```python
from build123d import *

# Parameters (mm, degrees)
SKETCH1_W           = 450
SKETCH1_H           = 45
BOSS_EXTRUDE1_DEPTH = 2
SKETCH2_R           = 1.5
CUT_EXTRUDE1_DEPTH  = 227.131046077
SKETCH3_R           = 2.5
CUT_EXTRUDE2_DEPTH  = 227.131046077
SKETCH4_R           = 10
CUT_EXTRUDE3_DEPTH  = 10


with BuildPart() as part:
    # Sketch1 → Boss-Extrude1 (new body)
    with BuildSketch(Plane.XY):
        Rectangle(SKETCH1_W, SKETCH1_H)
    extrude(amount=BOSS_EXTRUDE1_DEPTH)

    # Sketch2 → Cut-Extrude1 (cut, through all)
    with BuildSketch(Plane.XY.offset(2)):
        with Locations((-50.0375, -8.55)):
            Circle(SKETCH2_R)
        with Locations((-25.0375, -8.55)):
            Circle(SKETCH2_R)
        with Locations((-11.2375, -8.55)):
            Circle(SKETCH2_R)
        with Locations((13.7625, -8.55)):
            Circle(SKETCH2_R)
        with Locations((27.5625, -8.55)):
            Circle(SKETCH2_R)
        with Locations((52.5625, -8.55)):
            Circle(SKETCH2_R)
        with Locations((-88.8375, -8.55)):
            Circle(SKETCH2_R)
        with Locations((-63.8375, -8.55)):
            Circle(SKETCH2_R)
        with BuildLine():
            Line((-31.6625, -14.4), (-45.9375, -14.4))
            ThreePointArc((-45.9375, -14.4), (-46.644606781, -14.107106781), (-46.9375, -13.4))
            Line((-46.9375, -13.4), (-46.9375, -3.7))
            ThreePointArc((-46.9375, -3.7), (-46.586028137, -2.851471863), (-45.7375, -2.5))
            Line((-45.7375, -2.5), (-31.8625, -2.5))
            ThreePointArc((-31.8625, -2.5), (-29.22852724, -3.59102724), (-28.1375, -6.225))
            Line((-28.1375, -6.225), (-28.1375, -10.875))
            ThreePointArc((-28.1375, -10.875), (-29.169948596, -13.367551404), (-31.6625, -14.4))
        make_face()
        with BuildLine():
            Line((7.1375, -14.4), (-7.1375, -14.4))
            ThreePointArc((-7.1375, -14.4), (-7.844606781, -14.107106781), (-8.1375, -13.4))
            Line((-8.1375, -13.4), (-8.1375, -3.7))
            ThreePointArc((-8.1375, -3.7), (-7.786028137, -2.851471863), (-6.9375, -2.5))
            Line((-6.9375, -2.5), (6.9375, -2.5))
            ThreePointArc((6.9375, -2.5), (9.57147276, -3.59102724), (10.6625, -6.225))
            Line((10.6625, -6.225), (10.6625, -10.875))
            ThreePointArc((10.6625, -10.875), (9.630051404, -13.367551404), (7.1375, -14.4))
        make_face()
        with BuildLine():
            Line((45.9375, -14.4), (31.6625, -14.4))
            ThreePointArc((31.6625, -14.4), (30.955393219, -14.107106781), (30.6625, -13.4))
            Line((30.6625, -13.4), (30.6625, -3.7))
            ThreePointArc((30.6625, -3.7), (31.013971863, -2.851471863), (31.8625, -2.5))
            Line((31.8625, -2.5), (45.7375, -2.5))
            ThreePointArc((45.7375, -2.5), (48.37147276, -3.59102724), (49.4625, -6.225))
            Line((49.4625, -6.225), (49.4625, -10.875))
            ThreePointArc((49.4625, -10.875), (48.430051404, -13.367551404), (45.9375, -14.4))
        make_face()
        with BuildLine():
            Line((-70.4625, -14.4), (-84.7375, -14.4))
            ThreePointArc((-84.7375, -14.4), (-85.444606781, -14.107106781), (-85.7375, -13.4))
            Line((-85.7375, -13.4), (-85.7375, -3.7))
            ThreePointArc((-85.7375, -3.7), (-85.386028137, -2.851471863), (-84.5375, -2.5))
            Line((-84.5375, -2.5), (-70.6625, -2.5))
            ThreePointArc((-70.6625, -2.5), (-68.02852724, -3.59102724), (-66.9375, -6.225))
            Line((-66.9375, -6.225), (-66.9375, -10.875))
            ThreePointArc((-66.9375, -10.875), (-67.969948596, -13.367551404), (-70.4625, -14.4))
        make_face()
    extrude(amount=-CUT_EXTRUDE1_DEPTH, mode=Mode.SUBTRACT)

    # Sketch3 → Cut-Extrude2 (cut, through all)
    with BuildSketch(Plane.XY.offset(2)):
        with Locations((-215, 0)):
            Circle(SKETCH3_R)
        with Locations((215, 0)):
            Circle(SKETCH3_R)
        with Locations((-194, 12.495407459)):
            Circle(SKETCH3_R)
        with Locations((194, 12.495407459)):
            Circle(SKETCH3_R)
        with Locations((0, 12.5)):
            Circle(SKETCH3_R)
    extrude(amount=-CUT_EXTRUDE2_DEPTH, mode=Mode.SUBTRACT)

    # Sketch4 → Cut-Extrude3 (cut)
    with BuildSketch(Plane.XY.offset(2)):
        with Locations((-194, -8.55)):
            Circle(SKETCH4_R)
        with Locations((194, -8.55)):
            Circle(SKETCH4_R)
    extrude(amount=-CUT_EXTRUDE3_DEPTH, mode=Mode.SUBTRACT)


solid = part.part
```
Could you check a few things on this model? Use its own coordinates, in mm. Give positions to 0.01 mm unless a question says otherwise; leave off trailing zeros. Use one line per item in the form item = value.
1. I want a section at A-A (z = 1.2). Give the number of separate pieces and of enclosed holes in the cut face, and give its area (3 significant figures).
Response values:
separate_pieces = 1
enclosed_holes = 19
area = 18,600 mm²
2. Thinking about a two-plate mould opening in X: for faces 1 (the face through (-184.763, -12.38, 1.014)), 2 (the face through (-3, 0, 0)), 3 (the face through (203.237, -12.38, 1.014)), which applies, released by +X, released by -X, zero draft, split by the parting line, or undercut?
Response values:
face_1 = undercut
face_2 = zero draft
face_3 = undercut
3. I'm going to push a flat-ended pin straight in: pin 1 Ø4 at (x, y) = (194, 12.5) entering from +Z (3 decimals). Where does the tip first touch, or does it pass through?
Response values:
pin_1 = through
4. I need wall thicknesses on probe 1 along Y at (x, z) = (194, 1.45); probe 2 along X at (y, z) = (-15, 0.7); probe 3 along Y at (x, z) = (191, 1.6). Which ranges of each line are inside material? Lowest first, please.
Response values:
probe_1 = -22.5 to -18.55, 1.45 to 10, 15 to 22.5
probe_2 = -225 to -201.64, -186.36 to 186.36, 201.64 to 225
probe_3 = -22.5 to -18.09, 0.99 to 22.5
